Autodesk Fusion 360 part; units mm, degrees
sketch "Sketch1" plane through (0, 0, 0) normal (0, 0, 1) x (1, 0, 0)
  circle A0 centre (0, 0) radius 1.75
  circle A1 centre (-31, 0) radius 1.75
  line L0 (-27, -2) -> (-4, -2)
  line L1 (-27, 2) -> (-3.4641, 2)
  arc A2 (-27.8, 2.4) -> (-27.8, -2.4) centre (-31, 0) ccw
  arc A3 (-3.2, -2.4) -> (-3.4641, 2) centre (0, 0) ccw
  arc A4 (-27, -2) -> (-27.8, -2.4) centre (-27, -3) ccw
  arc A5 (-27.8, 2.4) -> (-27, 2) centre (-27, 3) ccw
  arc A6 (-3.2, -2.4) -> (-4, -2) centre (-4, -3) ccw
  point P0 (-31, 0)
  dimension "d7" = 8
  dimension "d8" = 3.5
  dimension "d9" = 8
  dimension "d10" = 3.5
  dimension "d11" = 1
  dimension "d12" = 1
  dimension "d13" = 1
extrude "Extrude1" add sketch "Sketch1" along normal blind 4
Source: CAD feature listing. Evaluate the final solid. Frame: model axes, mm. A direction names the side the tool comes from. Round coordinates to 2 decimals unless told otherwise and drop trailing zeros. Loops run counter-clockwise (first coordinate to the right, second up) from the corner with the lowest first, then second, coordinate; pieces in that order, holes last.
Q1. Section C-C, the plane z = 1.3. Return loops of the section in (x, y).
Q2. Access query for faces 3 (the face through (-27.44, 2.1, 1.97)), 4 (the face through (-32.75, -0.08, 1.97)), 5 (the face through (-16, -2, 2)). Directions: +Z, -Z, +X, -X, +Y, -Y. A direction counts if a zero-diameter tool reaches every point of the face in a straight line with its end or side. Return the directions, or none.
Q3. First-contact query: P1, Ø3, axis at x = -31, y = 0, coming from the -Z side; P2, Ø1.2, axis at x = -20.5, z = 2, coming from the -Y side. Flat tips, straight axial feed; report the tip coordinate or a pass-through.
Q4. Mould query, pull axis X, two halves, no side actions, for faces 1 (the face through (-15, 2, 2)), 2 (the face through (-16, 0, 4)). Classes: pulls with the +X half, pulls with the -X half, needs draft (parallel to the pull), parting line crosses it, or undercut.
Q5. Section A-A, the plane y = 0. Return loops of the section in (x, z), plus the area to 3 significant figures.
Q6. Ray query, line 1 (Y direction, x = -31, z = 2); line 2 (X direction, y = -0.75, z = 0.8); line 3 (X direction, y = -0.5, z = 1.9). Return the intervals inside material, ascending.
Q7. Section D-D, the plane x = -8. Return loops of the section in (y, z), plus the area to 3 significant figures.
Q8. Section B-B, the plane x = 0. Return loops of the section in (y, z).
Solutions:
1. outline: (-27.8, -2.4) arc R1 cw to (-27, -2) - (-4, -2) arc R1 cw to (-3.2, -2.4) arc R4 ccw (long way) to (-3.46, 2) - (-27, 2) arc R1 cw to (-27.8, 2.4) arc R4 ccw (long way) to start; hole circle Ø3.5 at (-31, 0); hole circle Ø3.5 at (0, 0)
2. face 3: +Z, -Z, +Y
2. face 4: +Z, -Z
2. face 5: +Z, -Z, -Y
3. P1: passes through
3. P2: stops at y = -2
4. face 1: undercut
4. face 2: needs draft
5. outline: (-35, 0) - (-32.75, 0) - (-32.75, 4) - (-35, 4) - close; (-29.25, 0) - (-1.75, 0) - (-1.75, 4) - (-29.25, 4) - close; (1.75, 0) - (4, 0) - (4, 4) - (1.75, 4) - close
5. area: 128 mm2
6. line 1: y = -4 to -1.75, 1.75 to 4
6. line 2: x = -34.93 to -32.58, -29.42 to -1.58, 1.58 to 3.93
6. line 3: x = -34.97 to -32.68, -29.32 to -1.68, 1.68 to 3.97
7. outline: (-2, 0) - (2, 0) - (2, 4) - (-2, 4) - close
7. area: 16.0 mm2
8. outline: (-4, 0) - (-1.75, 0) - (-1.75, 4) - (-4, 4) - close; (1.75, 0) - (4, 0) - (4, 4) - (1.75, 4) - close
